The listing builds one solid part. Answer for the finished solid, in the listing's coordinates (mm). Face numbers are marked on the shaded views. Round coordinates to 2 decimals unless told otherwise and drop trailing zeros. Order: outer loops, then holes, each group sorted by start corner. A loop starts at its lowest first (then second) coordinate and runs counter-clockwise, first axis right, second up. Notation, with made-up numbers: (62.5, 45) -> (89.5, 45) arc R23 cw to (89.5, 60) -> close; hole circle Ø8 at (44, 20.5). An arc over 180 degrees is marked (long way). Return JSON: item names as keys, results as strings. Group by question number.
(1) Each of these flat-tipped pins is pushed along its axis until it touches: pin 1 (3 mm diameter, centred on x = 11.5, z = -3, fed in from -Y); pin 2 (6 mm diameter, centred on x = -5, z = 7.5, fed in from +Y); pin 3 (12 mm diameter, centred on x = -11, z = -11, fed in from +Y); pin 4 (2 mm diameter, centred on y = 1.5, z = 4, fed in from -X). Where does it stop, or does it pass through?
(2) The part is cut by section D-D (z = 12). Determine the outline of the cut face in (x, y), plus the area to 3 significant figures.
(3) The part is cut by section A-A (z = 0). Count the separate pieces of the cut face and the enclosed holes in it, plus the area to 3 significant figures.
(4) Consider line 1 (Z direction, x = -9, y = 4.9); line 2 (Z direction, x = 13, y = 5); line 3 (X direction, y = 0.4, z = -1). Determine where each line is inside the solid, lowest interval first. Write a range as [from, to].
(5) Determine the mould class of the marked faces 1, 2 and 3 for opening direction X: +X half, -X half, draft (parallel to the pull), parting line (faces both ways), or undercut.
(6) The part is cut by section B-B (y = 0.7). Determine the outline of the cut face in (x, z), plus the area to 3 significant figures.
from build123d import *

# Parameters (mm, degrees)
SKETCH1_R           = 4.064
SKETCH1_R_2         = 2.794
BOSS_EXTRUDE1_DEPTH = 3.302
SKETCH2_R           = 0.62500002
SKETCH2_R_2         = 4.064
SKETCH2_R_3         = 2.794
BOSS_EXTRUDE2_DEPTH = 1.87000007
SKETCH6_R           = 1.449999894
CUT_EXTRUDE6_DEPTH  = 23.164493782
SKETCH7_R           = 3.555000002
SKETCH7_R_2         = 2.819999948
BOSS_EXTRUDE3_DEPTH = 0.470000076


with BuildPart() as part:
    # Sketch1 → Boss-Extrude1 (new body)
    with BuildSketch(Plane(origin=(0, 0, 0), x_dir=(1, 0, 0), z_dir=(0, 1, 0))):
        with Locations(Location((0, 0, 0), (0, 0, 90))):
            Circle(SKETCH1_R)
        with Locations(Location((0, 0, 0), (0, 0, 90))):
            Circle(SKETCH1_R_2, mode=Mode.SUBTRACT)
    extrude(amount=BOSS_EXTRUDE1_DEPTH)

    # Sketch2 → Boss-Extrude2 (add)
    # profile 1 of 3: a face of its own
    with BuildSketch(Plane(origin=(0, 3.302, 0), x_dir=(1, 0, 0), z_dir=(0, 1, 0))):
        with BuildLine():
            ThreePointArc((-6.598095019, 3.184398134), (-4.342465091, 4.342465091), (-3.184398134, 6.598095019))
            Line((-3.184398134, 6.598095019), (-1.973411671, 13.950499547))
            ThreePointArc((-1.973411671, 13.950499547), (-1e-09, 15.239999998), (1.973411671, 13.950499548))
            Line((1.973411671, 13.950499548), (3.184398134, 6.598095019))
            ThreePointArc((3.184398134, 6.598095019), (4.342465091, 4.342465091), (6.598095019, 3.184398134))
            Line((6.598095019, 3.184398134), (13.950499547, 1.973411671))
            ThreePointArc((13.950499547, 1.973411671), (15.239999998, 1e-09), (13.950499548, -1.973411671))
            Line((13.950499548, -1.973411671), (6.598095019, -3.184398134))
            ThreePointArc((6.598095019, -3.184398134), (4.342465091, -4.342465091), (3.184398134, -6.598095019))
            Line((3.184398134, -6.598095019), (1.973411671, -13.950499547))
            ThreePointArc((1.973411671, -13.950499547), (1e-09, -15.239999998), (-1.973411671, -13.950499548))
            Line((-1.973411671, -13.950499548), (-3.184398134, -6.598095019))
            ThreePointArc((-3.184398134, -6.598095019), (-4.342465091, -4.342465091), (-6.598095019, -3.184398134))
            Line((-6.598095019, -3.184398134), (-13.950499547, -1.973411671))
            ThreePointArc((-13.950499547, -1.973411671), (-15.239999998, -1e-09), (-13.950499548, 1.973411671))
            Line((-13.950499548, 1.973411671), (-6.598095019, 3.184398134))
        make_face()
        with Locations(Location((-13.500466522, 0, 0), (0, 0, 270))):
            Circle(SKETCH2_R, mode=Mode.SUBTRACT)
        with Locations(Location((-10.500466426, 0, 0), (0, 0, 270))):
            Circle(SKETCH2_R, mode=Mode.SUBTRACT)
        with Locations(Location((-7.50046633, 0, 0), (0, 0, 270))):
            Circle(SKETCH2_R, mode=Mode.SUBTRACT)
        with Locations(Location((13.500466522, 0, 0), (0, 0, 270))):
            Circle(SKETCH2_R, mode=Mode.SUBTRACT)
        with Locations(Location((10.500466426, 0, 0), (0, 0, 270))):
            Circle(SKETCH2_R, mode=Mode.SUBTRACT)
        with Locations(Location((7.50046633, 0, 0), (0, 0, 270))):
            Circle(SKETCH2_R, mode=Mode.SUBTRACT)
        with Locations(Location((0, 7.50046633, 0), (0, 0, 270))):
            Circle(SKETCH2_R, mode=Mode.SUBTRACT)
        with Locations(Location((0, 10.500466426, 0), (0, 0, 270))):
            Circle(SKETCH2_R, mode=Mode.SUBTRACT)
        with Locations(Location((0, 13.500466522, 0), (0, 0, 270))):
            Circle(SKETCH2_R, mode=Mode.SUBTRACT)
        with Locations(Location((0, -13.500466522, 0), (0, 0, 270))):
            Circle(SKETCH2_R, mode=Mode.SUBTRACT)
        with Locations(Location((0, -10.500466426, 0), (0, 0, 270))):
            Circle(SKETCH2_R, mode=Mode.SUBTRACT)
        with Locations(Location((0, -7.50046633, 0), (0, 0, 270))):
            Circle(SKETCH2_R, mode=Mode.SUBTRACT)
        with Locations(Location((0, 0, 0), (0, 0, 90))):
            Circle(SKETCH2_R_2, mode=Mode.SUBTRACT)
    # profile 2 of 3: a face of its own
    with BuildSketch(Plane(origin=(0, 3.302, 0), x_dir=(1, 0, 0), z_dir=(0, 1, 0))):
        with Locations(Location((0, 0, 0), (0, 0, 90))):
            Circle(SKETCH2_R_2)
        with Locations(Location((0, 0, 0), (0, 0, 90))):
            Circle(SKETCH2_R_3, mode=Mode.SUBTRACT)
    # profile 3 of 3: a face of its own
    with BuildSketch(Plane(origin=(0, 3.302, 0), x_dir=(1, 0, 0), z_dir=(0, 1, 0))):
        with Locations(Location((0, 0, 0), (0, 0, 90))):
            Circle(SKETCH2_R_3)
    extrude(amount=BOSS_EXTRUDE2_DEPTH)

    # Sketch6 → Cut-Extrude6 (cut, through all)
    with BuildSketch(Plane(origin=(0, 5.17200007, 0), x_dir=(1, 0, 0), z_dir=(0, 1, 0))):
        with Locations(Location((0, 0, 0), (0, 0, 270))):
            Circle(SKETCH6_R)
    extrude(amount=-CUT_EXTRUDE6_DEPTH, mode=Mode.SUBTRACT)

    # Sketch7 → Boss-Extrude3 (add)
    with BuildSketch(Plane(origin=(0, 5.17200007, 0), x_dir=(1, 0, 0), z_dir=(0, 1, 0))):
        with Locations(Location((0, 0, 0), (0, 0, 270))):
            Circle(SKETCH7_R)
        with Locations(Location((0, 0, 0), (0, 0, 270))):
            Circle(SKETCH7_R_2, mode=Mode.SUBTRACT)
    extrude(amount=BOSS_EXTRUDE3_DEPTH)


solid = part.part
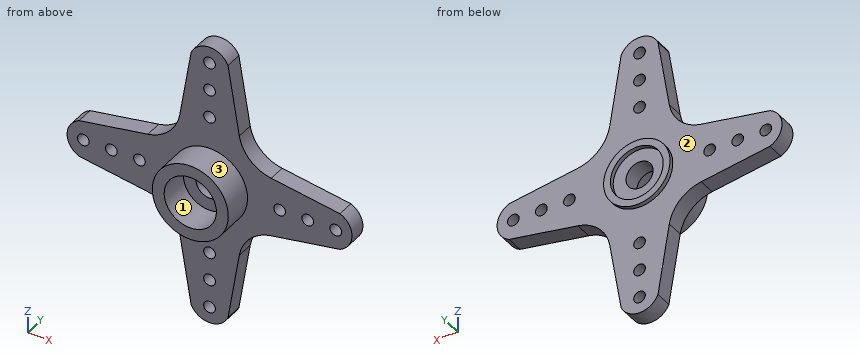
Answer below:
{
 "1": {"pin 1": "stops at y = 3.3", "pin 2": "stops at y = 5.17", "pin 3": "passes through", "pin 4": "stops at x = -2.74"},
 "2": {"outline": "(-2.29, 3.3) -> (2.29, 3.3) -> (2.29, 5.17) -> (-2.29, 5.17) -> close", "area": "8.58 mm²"},
 "3": {"separate pieces": "8", "enclosed holes": "0", "area": "46.6 mm²"},
 "4": {"line 1": "z = [-2.79, 2.79]", "line 2": "z = [-2.13, -0.37], [0.37, 2.13]", "line 3": "x = [-3.94, -2.61], [2.61, 3.94]"},
 "5": {"face 1": "undercut", "face 2": "draft", "face 3": "parting line"},
 "6": {"outline": "circle Ø8.13 at (0, 0); hole circle Ø5.59 at (0, 0)", "area": "27.4 mm²"}
}
